Input: part model. Units: mm. Frame: model coordinates. Round coordinates to 2 decimals unless told otherwise and drop trailing zeros. Write each loop counter-clockwise with the first axis right and the second up, starting at its lowest first coordinate (ties: lowest second). Pieces come first, ordered by that corner, then holes. Notation, with made-up numbers: (41.25, 14.5) -> (94.25, 14.5) arc R30 ccw to (94.25, 40.5) -> close; hole circle Ø10 at (-2, -18). An arc over 180 degrees is marked (long way). Write item = value, one per line.
```python
from build123d import *

# Parameters (mm, degrees)
F1_DEPTH = 1298.956
F2_W     = 113.868274
F2_H     = 929.21856
F3_DEPTH = 23.877


with BuildPart() as f1:
    # F0 (on Front) → F1 (new body, symmetric)
    with BuildSketch(Plane.XZ):
        with BuildLine():
            Line((63.246, 11.938), (-63.246, 11.938))
            ThreePointArc((-63.246, 11.938), (-66.658497, 10.524497), (-68.072, 7.112))
            Line((-68.072, 7.112), (-68.072, -7.112))
            ThreePointArc((-68.072, -7.112), (-66.658497, -10.524497), (-63.246, -11.938))
            Line((-63.246, -11.938), (63.246, -11.938))
            ThreePointArc((63.246, -11.938), (66.658497, -10.524497), (68.072, -7.112))
            Line((68.072, -7.112), (68.072, 7.112))
            ThreePointArc((68.072, 7.112), (66.658497, 10.524497), (63.246, 11.938))
        make_face()
    extrude(amount=F1_DEPTH, both=True)

    # F2 (on face) → F3 (cut, through all)
    with BuildSketch(Plane.XY.offset(11.938)):
        with Locations((56.934137, 976.16528)):
            Rectangle(F2_W, F2_H)
    extrude(amount=-F3_DEPTH, mode=Mode.SUBTRACT)


solid = f1.part
```
1) Cut plane A-A (z = 2.5). Return the cut outline in (x, y).
Solutions:
outline = (-68.07, -1298.96) -> (68.07, -1298.96) -> (68.07, 511.56) -> (0, 511.56) -> (0, 1298.96) -> (-68.07, 1298.96) -> close
2) Cut plane C-C (x = 30). Return the cut outline in (y, z).
Solutions:
outline = (-1298.96, -11.94) -> (511.56, -11.94) -> (511.56, 11.94) -> (-1298.96, 11.94) -> close
3) Cut plane B-B (y = 1068). Return the cut outline in (x, z), and give its area (3 significant figures).
Solutions:
outline = (-68.07, -7.11) arc R4.83 ccw to (-63.25, -11.94) -> (0, -11.94) -> (0, 11.94) -> (-63.25, 11.94) arc R4.83 ccw to (-68.07, 7.11) -> close
area = 1,620 mm^2
4) Draft query along Z for faces 1 (the face through (-1, -307, -11.938)), 2 (the face through (1, -307, 11.938)). Return one class per face: +Z half, -Z half, draft (parallel to the pull), parting line (faces both ways), or undercut.
Solutions:
face_1 = -Z half
face_2 = +Z half
5) First-contact query: P1, Ø12, axis at x = 48.5, z = -3.5, coming from the +Y side. Flat tip, straight axial feed; report the tip coordinate or a pass-through.
Solutions:
P1 = 511.56
6) Line query: L1, parallel to Y at x = 13.5, z = 10.25; L2, parallel to X at y = 972, z = 7; L3, parallel to X at y = 118.5, z = -7.5. Output: solid intervals per line, ascending. Write a range as from..to.
Solutions:
L1 = -1298.96..511.56
L2 = -68.07..0
L3 = -68.06..68.06
